from build123d import *

# Parameters (mm, degrees)
F0_W     = 550
F0_H     = 550
F1_DEPTH = 50
F2_R     = 15
F3_W     = 300
F3_H     = 200
F4_DEPTH = 20


with BuildPart() as f1:
    # F0 (on Top) → F1 (new body)
    with BuildSketch(Plane.XY):
        Rectangle(F0_W, F0_H)
    extrude(amount=F1_DEPTH)

    # F2
    f2_edges = [f1.edges().sort_by_distance(p)[0] for p in [
        (0, -275, 50),
        (275, 0, 50),
        (0, 275, 50),
        (-275, 0, 50),
        (275, -275, 25),
        (275, 275, 25),
        (-275, 275, 25),
        (-275, -275, 25),
    ]]
    fillet(f2_edges, radius=F2_R)

    # F3 (on face) → F4 (cut)
    with BuildSketch(Plane.XY.offset(50)):
        Rectangle(F3_W, F3_H)
    extrude(amount=-F4_DEPTH, mode=Mode.SUBTRACT)


solid = f1.part
Design review of the part built by this model. Coordinates are the model's own, in mm. A direction names the side the tool comes from. Round coordinates to 2 decimals unless told otherwise and drop trailing zeros. Order: outer loops, then holes, each group sorted by start corner. A loop starts at its lowest first (then second) coordinate and runs counter-clockwise, first axis right, second up.
1) For L1, parallel to X at y = 2, z = 34; L2, parallel to X at y = -41.5, z = 41; L3, parallel to Z at x = 28.5, y = -18, list the stretches that pass through material, from the lowest coordinate up.
The answers:
L1: x = -275 to -150, 150 to 275
L2: x = -273.75 to -150, 150 to 273.75
L3: z = 0 to 30
2) Machinability: for faces 1 (the flat face through (-4, 119, 50)), 2 (the flat face through (-2, 100, 40)), which of the approach directions +Z, -Z, +X, -X, +Y, -Y give a long, thin tool a straight path to every point of the face, cutting with its end or side? Answer none if there is none.
The answers:
face 1: +Z, +X, -X, +Y, -Y
face 2: +Z
3) Draft analysis for pull direction X (two halves, no side actions). For faces 3 (the cylindrical face through (3.64, 270.72, 45.49)), 4 (the cylindrical face through (270.72, 270.49, 17.74)), 5 (the cylindrical face through (-270.72, 270.49, 17.74)), 6 (the flat face through (-2, 1, 30)), state which applies: released by +X, released by -X, zero draft, split by the parting line, or undercut.
The answers:
face 3: zero draft
face 4: released by +X
face 5: released by -X
face 6: undercut
4) Clearance check with flat-ended pins moving along their axes: pin 1 Ø3 at (y, z) = (13.5, 43.5) entering from +X; pin 2 Ø6 at (y, z) = (21.5, 41.5) entering from +X; pin 3 Ø10 at (x, z) = (29.5, 41.5) entering from +Y. State where each tip first meets the part, or that it passes through.
The answers:
pin 1: stops at x = 273.27
pin 2: stops at x = 274.59
pin 3: stops at y = 274.92
5) Consider section A-A (x = -117.5). State the section outline as (y, z) points.
The answers:
outline: (-275, 0) - (275, 0) - (275, 35) arc R15 ccw to (260, 50) - (100, 50) - (100, 30) - (-100, 30) - (-100, 50) - (-260, 50) arc R15 ccw to (-275, 35) - close
